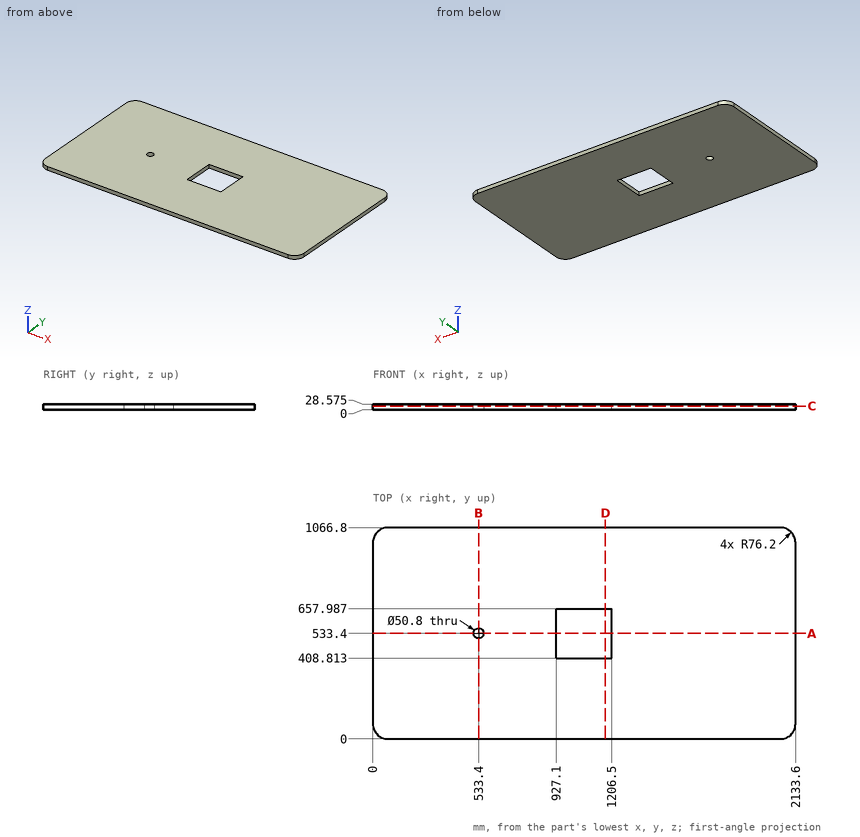
Here's the drawing with two shaded views (mm, measured from the low corner). I have some questions. Round coordinates to 2 decimals unless told otherwise and drop trailing zeros. Write each loop counter-clockwise with the first axis right and the second up, starting at its lowest first coordinate (ties: lowest second). Pieces come first, ordered by that corner, then holes.
(1) Suppose I cut it at C-C on z = 17.25. Write out the boundary of the cut face in (x, y).
Findings below:
outline: (0, 76.2) arc R76.2 ccw to (76.2, 0) - (2057.4, 0) arc R76.2 ccw to (2133.6, 76.2) - (2133.6, 990.6) arc R76.2 ccw to (2057.4, 1066.8) - (76.2, 1066.8) arc R76.2 ccw to (0, 990.6) - close; hole circle Ø50.8 at (533.4, 533.4); hole (927.1, 408.81) - (1206.5, 408.81) - (1206.5, 657.99) - (927.1, 657.99) - close
(2) Suppose I cut it at B-B on x = 533.4. Write out the boundary of the cut face in (y, z) (3 decimals).
Findings below:
outline: (0, 0) - (508, 0) - (508, 28.575) - (0, 28.575) - close; (558.8, 0) - (1066.8, 0) - (1066.8, 28.575) - (558.8, 28.575) - close
(3) Suppose I cut it at D-D on x = 1174. Write out the boundary of the cut face in (y, z) (3 decimals), and give its area (3 significant figures).
Findings below:
outline: (0, 0) - (408.813, 0) - (408.813, 28.575) - (0, 28.575) - close; (657.987, 0) - (1066.8, 0) - (1066.8, 28.575) - (657.987, 28.575) - close
area: 23,400 mm2
(4) If I drill on probe 1 along Y at (x, z) = (533.4, 19); probe 2 along X at (y, z) = (639, 15.5), over which ranges is the centre line in solid material (lowest first)?
Findings below:
probe 1: y = 0 to 508, 558.8 to 1066.8
probe 2: x = 0 to 927.1, 1206.5 to 2133.6
(5) Suppose I cut it at A-A on y = 533.4. Write out the boundary of the cut face in (x, z) (3 decimals).
Findings below:
outline: (0, 0) - (508, 0) - (508, 28.575) - (0, 28.575) - close; (558.8, 0) - (927.1, 0) - (927.1, 28.575) - (558.8, 28.575) - close; (1206.5, 0) - (2133.6, 0) - (2133.6, 28.575) - (1206.5, 28.575) - close
